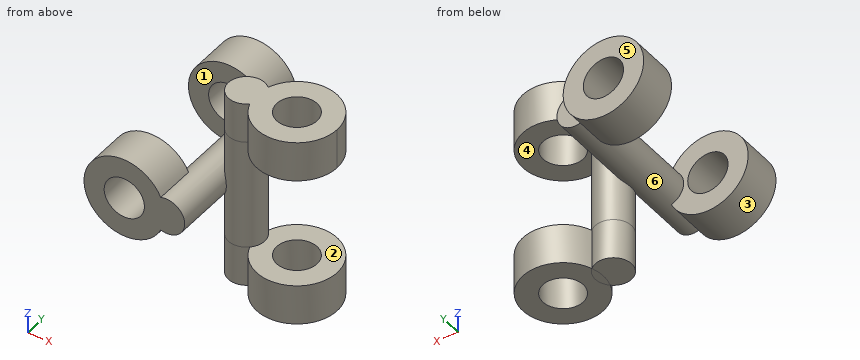
from build123d import *

# Parameters (mm, degrees)
SKETCH_1_R             = 2
SKETCH_1_R_2           = 1
EXTRUDE_1_DEPTH        = 2
EXTRUDE_1_2_DEPTH      = 7.5
EXTRUDE_1_2_DEPTH_BACK = 1
SKETCH_2_R             = 0.9
SKETCH_3_R             = 2
SKETCH_3_R_2           = 1
EXTRUDE_2_DEPTH        = 2
SKETCH_7_R             = 0.5
EXTRUDE_4_DEPTH        = 2
EXTRUDE_7_DEPTH        = 2.75
EXTRUDE_7_DEPTH_BACK   = 2.75
SKETCH_11_R            = 0.9
SKETCH_12_R            = 2
SKETCH_12_R_2          = 1
EXTRUDE_5_DEPTH        = 2
EXTRUDE_START          = 2
SKETCH_13_R            = 2
SKETCH_13_R_2          = 1
EXTRUDE_6_DEPTH        = 2
SKETCH_15_R            = 0.9
EXTRUDE_8_DEPTH        = 2
SKETCH_16_R            = 0.9
EXTRUDE_9_DEPTH        = 2


with BuildPart() as part:
    # Sketch 1 → Extrude 1 (new body)
    with BuildSketch(Plane(origin=(0, 0, 0), x_dir=(1, 0, 0), z_dir=(0, 1, 0))):
        Circle(SKETCH_1_R)
        Circle(SKETCH_1_R_2, mode=Mode.SUBTRACT)
    extrude(amount=EXTRUDE_1_DEPTH)

    # Sketch 2 → Extrude 1 2 (add, two sides: drawn at the far end of the back side and taken through both)
    with BuildSketch(Plane.XZ.offset(-EXTRUDE_1_2_DEPTH_BACK)):
        with Locations(Location((2.1, 0, 0), (0, 0, 270))):
            Circle(SKETCH_2_R)
    extrude(amount=EXTRUDE_1_2_DEPTH + EXTRUDE_1_2_DEPTH_BACK)

    # Sketch 3 → Extrude 2 (add)
    with BuildSketch(Plane.XZ.offset(7.5)):
        with Locations(Location((0, 0, 0), (0, 0, 334.791234703))):
            Circle(SKETCH_3_R)
        with Locations(Location((0, 0, 0), (0, 0, 90))):
            Circle(SKETCH_3_R_2, mode=Mode.SUBTRACT)
    extrude(amount=-EXTRUDE_2_DEPTH)

    # Sketch 7 → Extrude 4 (add)
    with BuildSketch(Plane(origin=(1.877338573, 0, 0), x_dir=(0, 0, -1), z_dir=(1, 0, 0))):
        with Locations(Location((0, -3.75, 0), (0, 0, 180))):
            Circle(SKETCH_7_R)
    extrude(amount=EXTRUDE_4_DEPTH)

    # Sketch 11 → Extrude 7 (add, two sides: drawn at the far end of the back side and taken through both)
    with BuildSketch(Plane.XY.offset(-EXTRUDE_7_DEPTH_BACK)):
        with Locations((3.477338573, -3.75)):
            Circle(SKETCH_11_R)
    extrude(amount=EXTRUDE_7_DEPTH + EXTRUDE_7_DEPTH_BACK)

    # Sketch 12 → Extrude 5 (add)
    with BuildSketch(Plane.XY.offset(2.75)):
        with Locations((5.977338573, -3.75)):
            Circle(SKETCH_12_R)
        with Locations((5.977338573, -3.75)):
            Circle(SKETCH_12_R_2, mode=Mode.SUBTRACT)
    extrude(amount=EXTRUDE_5_DEPTH)

    # Sketch 13 → Extrude 6 (add)
    with BuildSketch(Plane(origin=(0, 0, -2.75), x_dir=(-1, 0, 0), z_dir=(0, 0, -1)).offset(EXTRUDE_START)):
        with Locations((-5.977338573, -3.75)):
            Circle(SKETCH_13_R)
        with Locations((-5.977338573, -3.75)):
            Circle(SKETCH_13_R_2, mode=Mode.SUBTRACT)
    extrude(amount=-EXTRUDE_6_DEPTH)

    # Sketch 15 → Extrude 8 (add)
    with BuildSketch(Plane(origin=(0, 0, -2.75), x_dir=(-1, 0, 0), z_dir=(0, 0, -1))):
        with Locations(Location((-3.477338573, -3.75, 0), (0, 0, 227.156356956))):
            Circle(SKETCH_15_R)
    extrude(amount=EXTRUDE_8_DEPTH)

    # Sketch 16 → Extrude 9 (add)
    with BuildSketch(Plane.XY.offset(2.75).offset(EXTRUDE_START)):
        with Locations(Location((3.477338573, -3.75, 0), (0, 0, 312.843643044))):
            Circle(SKETCH_16_R)
    extrude(amount=-EXTRUDE_9_DEPTH)


solid = part.part
Check sheet for the modelled part. Datum: model origin and axes. Units: mm. Face numbers are marked on the shaded views. A direction names the side the tool comes from. Coordinates: 2 decimals unless noted, no trailing zeros. Write each loop counter-clockwise with the first axis right and the second up, starting at its lowest first coordinate (ties: lowest second). Pieces come first, ordered by that corner, then holes.
Item 1: Access from +Z, -Z, +X, -X, +Y, -Y to the whole of each face (thin tool, end or side, straight path). Record for the marked faces 5 and 6.
Numbers:
face 5: +Z, -Z, +X, -X, +Y
face 6: none
Item 2: Scan lines: probe 1 along Y at (x, z) = (0.25, 1.5); probe 2 along Z at (x, y) = (4.5, -3.25); probe 3 along X at (y, z) = (-6.35, 0). Record each from-to range of solid material in increasing order.
Numbers:
probe 1: y = -7.5 to -5.5, 0 to 2
probe 2: z = -4.75 to -2.75, 2.75 to 4.75
probe 3: x = -2 to -1, 1 to 3
Item 3: Cross-section at C-C on y = -2. Record the boundary of the cut face in (x, z).
Numbers:
outline: circle Ø1.8 at (2.1, 0); (5.01, -4.75) - (6.95, -4.75) - (6.95, -2.75) - (5.01, -2.75) - close; (5.01, 2.75) - (6.95, 2.75) - (6.95, 4.75) - (5.01, 4.75) - close
Item 4: Cross-section at A-A on x = 0. Record the boundary of the cut face in (y, z), then the cut area to 3 significant figures.
Numbers:
outline: (-7.5, -2) - (-5.5, -2) - (-5.5, -1) - (-7.5, -1) - close; (-7.5, 1) - (-5.5, 1) - (-5.5, 2) - (-7.5, 2) - close; (0, -2) - (2, -2) - (2, -1) - (0, -1) - close; (0, 1) - (2, 1) - (2, 2) - (0, 2) - close
area: 8.00 mm2
Item 5: Mould release check, pull along Z, two halves, no side actions. Record for the marked faces 1, 2, 3 and 4: released by +Z, released by -Z, zero draft, split by the parting line, or undercut.
Numbers:
face 1: zero draft
face 2: undercut
face 3: split by the parting line
face 4: undercut
Item 6: Cross-section at B-B on z = -0.25. Record the boundary of the cut face in (x, y), then the cut area to 3 significant figures.
Numbers:
outline: (-1.98, -7.5) - (-0.97, -7.5) - (-0.97, -5.5) - (-1.98, -5.5) - close; (-1.98, 0) - (-0.97, 0) - (-0.97, 2) - (-1.98, 2) - close; (0.97, -7.5) - (2.96, -7.5) - (2.96, -4.49) arc R0.9 ccw (long way) to (2.96, -3.01) - (2.96, 1) - (1.98, 1) - (1.98, 2) - (0.97, 2) - (0.97, 0) - (1.24, 0) - (1.24, -5.5) - (0.97, -5.5) - close
area: 22.7 mm2
Item 7: Cross-section at D-D on z = 3. Record the boundary of the cut face in (x, y).
Numbers:
outline: (4.09, -4.41) arc R2 ccw (long way) to (4.09, -3.09) arc R0.9 ccw (long way) to start; hole circle Ø2 at (5.98, -3.75)
Item 8: Depth check by flat-ended pin: pin 1 Ø4 at (y, z) = (-4.5, 0.5) entering from +X; pin 2 Ø3 at (x, y) = (5.98, -3.75) entering from -Z; pin 3 Ø0.6 at (x, z) = (2.5, -0.5) entering from +Y. Enter the tip coordinate at first touch or a pass-through.
Numbers:
pin 1: stops at x = 4.38
pin 2: stops at z = -4.75
pin 3: stops at y = 1
